Geometry check sheet. Reference: the model listing, model coordinates, mm. Coordinates: 2 decimals unless noted, no trailing zeros. Order: outer loops, then holes, each group sorted by start corner. A loop starts at its lowest first (then second) coordinate and runs counter-clockwise, first axis right, second up. Notation, with made-up numbers: (41.5, 28) - (62.5, 28) arc R32 cw to (62.5, 64) - close; hole circle Ø7 at (53.5, -34). An arc over 180 degrees is marked (long way). Put each result on its own line as item: value.
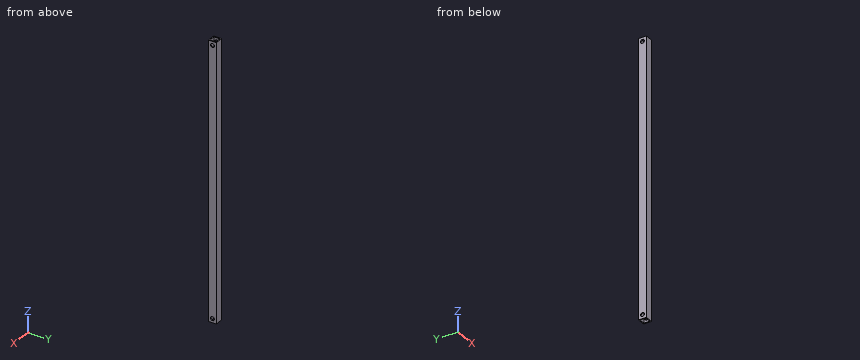
Autodesk Inventor part; units mm, degrees
ref_plane "YZ Plane" through (0, 0, 0) normal (1, 0, 0) x (0, 1, 0)
ref_plane "XZ Plane" through (0, 0, 0) normal (0, 1, 0) x (-1, 0, 0)
ref_plane "XY Plane" through (0, 0, 0) normal (0, 0, 1) x (1, 0, 0)
sketch "Sketch1" plane through (0, 0, 0) normal (0, 0, 1) x (1, 0, 0)
  line L0 (0, 0) -> (25.4, 0)
  line L1 (25.4, 0) -> (25.4, -25.4)
  line L2 (25.4, -25.4) -> (0, -25.4)
  line L3 (0, -25.4) -> (0, 0)
  dimension "d0" = 25.4
  dimension "d1" = 25.4
extrude "Extrusion1" add sketch "Sketch1" along normal blind 889
shell "Shell1" thickness 3.175 removed faces 2 at (8.4667, -8.4667, 0) at (8.4667, -8.4667, 889)
sketch "Sketch2" plane through (25.4, -25.4, 0) normal (1, 0, 0) x (0, 0, -1)
  circle A0 centre (-12.7, 12.7) radius 6.35
  line L0 (0, 25.4) -> (-889, 25.4)
  line L1 (0, 25.4) -> (0, 0)
  circle A1 centre (-876.3, 12.7) radius 6.35
  line L2 (-889, 0) -> (-889, 25.4)
  dimension "d5" = 12.7
  dimension "d6" = 12.7
  dimension "d7" = 12.7
  dimension "d10" = 12.7
  dimension "d11" = 12.7
  dimension "d12" = 12.7
extrude "Extrusion2" cut sketch "Sketch2" against normal blind 889
properties part number "Kermit Frame 16"
Q1. Thickness scan on L1, parallel to X at y = -4, z = 278 (3 decimals); L2, parallel to Y at x = 2.15, z = 12.7; L3, parallel to Y at x = 16.5, z = 449 (3 decimals). Record the ranges inside material, lowest first. Write a range as [from, to].
Answer block:
L1: x = [0, 3.175], [22.225, 25.4]
L2: y = [-25.4, -19.05], [-6.35, 0]
L3: y = [-25.4, -22.225], [-3.175, 0]
Q2. Section check A-A on x = 15.75. Record the boundary of the cut face in (y, z) (3 decimals).
Answer block:
outline: (-25.4, 0) - (-22.225, 0) - (-22.225, 889) - (-25.4, 889) - close; (-3.175, 0) - (0, 0) - (0, 889) - (-3.175, 889) - close
Q3. Section check B-B on y = -12.7. Record the boundary of the cut face in (x, z) (3 decimals).
Answer block:
outline: (0, 0) - (3.175, 0) - (3.175, 6.35) - (0, 6.35) - close; (0, 19.05) - (3.175, 19.05) - (3.175, 869.95) - (0, 869.95) - close; (0, 882.65) - (3.175, 882.65) - (3.175, 889) - (0, 889) - close; (22.225, 0) - (25.4, 0) - (25.4, 6.35) - (22.225, 6.35) - close; (22.225, 19.05) - (25.4, 19.05) - (25.4, 869.95) - (22.225, 869.95) - close; (22.225, 882.65) - (25.4, 882.65) - (25.4, 889) - (22.225, 889) - close
Q4. Section check C-C on z = 614. Record the boundary of the cut face in (x, y) (3 decimals), then the cut area to 3 significant figures.
Answer block:
outline: (0, -25.4) - (25.4, -25.4) - (25.4, 0) - (0, 0) - close; hole (3.175, -22.225) - (22.225, -22.225) - (22.225, -3.175) - (3.175, -3.175) - close
area: 282 mm^2
